Job drawing, mm, ordinate dimensions from the low corner. One solid piece. Round coordinates to 2 decimals unless told otherwise and drop trailing zeros. Loops run counter-clockwise (first coordinate to the right, second up) from the corner with the lowest first, then second, coordinate; pieces in that order, holes last.
1) Probe line 1 (Z direction, x = 3, y = 0.8); line 2 (X direction, y = 1.15, z = 57); line 3 (X direction, y = 1.2, z = 3). List the from-to ranges inside material, lowest first.
2) Drop a flat-ended pin along its axis: P1, Ø0.5, axis at x = 31, y = 0.5, coming from the -Z side. Give the stop position or say it passes through.
3) Band-saw the part on A-A, the plane y = 1. Write the cut outline in (x, z), then the cut area to 3 significant figures.
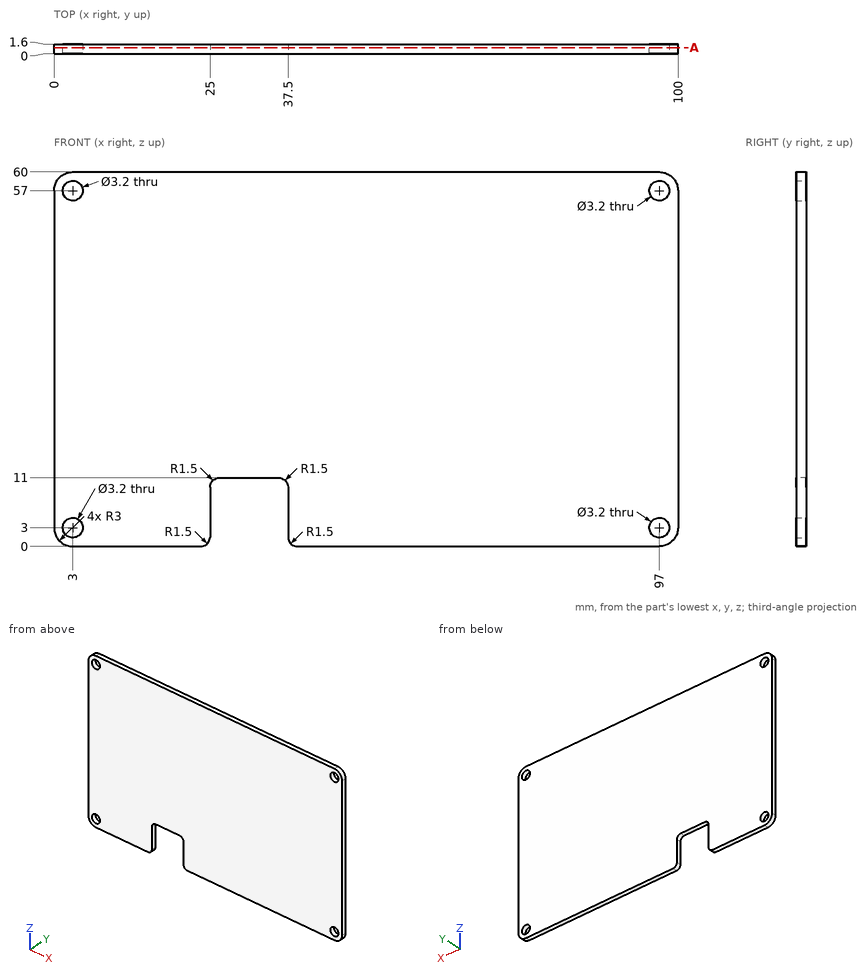
Reported:
1. line 1: z = 0 to 1.4, 4.6 to 55.4, 58.6 to 60
1. line 2: x = 0 to 1.4, 4.6 to 95.4, 98.6 to 100
1. line 3: x = 0 to 1.4, 4.6 to 25, 37.5 to 95.4, 98.6 to 100
2. P1: stops at z = 11
3. outline: (0, 3) arc R3 ccw to (3, 0) - (23.5, 0) arc R1.5 ccw to (25, 1.5) - (25, 9.5) arc R1.5 cw to (26.5, 11) - (36, 11) arc R1.5 cw to (37.5, 9.5) - (37.5, 1.5) arc R1.5 ccw to (39, 0) - (97, 0) arc R3 ccw to (100, 3) - (100, 57) arc R3 ccw to (97, 60) - (3, 60) arc R3 ccw to (0, 57) - close; hole circle Ø3.2 at (3, 3); hole circle Ø3.2 at (3, 57); hole circle Ø3.2 at (97, 3); hole circle Ø3.2 at (97, 57)
3. area: 5,820 mm2
